Can you work these out from the drawing? Everything is in mm from the part's minimum corner. A direction names the side the tool comes from. Round coordinates to 2 decimals unless told otherwise and drop trailing zeros. Write each loop counter-clockwise with the first axis right and the second up, starting at its lowest first coordinate (ties: lowest second). Pieces come first, ordered by that corner, then holes. Notation, with made-up numbers: (43.25, 80) -> (72.25, 80) arc R17 cw to (72.25, 94) -> close; hole circle Ø9 at (66, 76.25). An arc over 180 degrees is marked (long way). Write item = value, one per line. Start each with the question number.
1) Imagine slicing it at A-A, the plane y = 15. Please give me the cut outline in (x, z).
2) Imagine slicing it at C-C, the plane z = 36.5. Please give me the cut outline in (x, y).
3) If I drill on line 1 (Z direction, x = 5.5, y = 2.25); line 2 (Z direction, x = 10.25, y = 6.5); line 3 (Y direction, x = 16.25, z = 31.5), over which ranges is the centre line in solid material (lowest first)?
4) Imagine slicing it at B-B, the plane x = 15. Please give me the cut outline in (y, z).
5) Imagine slicing it at D-D, the plane x = 7.75. Please give me the cut outline in (y, z), then the cut area to 3 significant figures.
6) For the marked faces 1, 2 and 3, which set-ups out of +Z, -Z, +X, -X, +Y, -Y let a thin tool reach every point of the face, with its end or its side?
7) I'm going to push flat-ended pins straight in: pin 1 (1.2 mm diameter, centred on x = 8, z = 48, fed in from +Y); pin 2 (6 mm diameter, centred on x = 10.5, z = 15.5, fed in from -Y); pin 3 (12 mm diameter, centred on y = 18.5, z = 13.5, fed in from -X). Where does each tip first touch, or does it pass through?
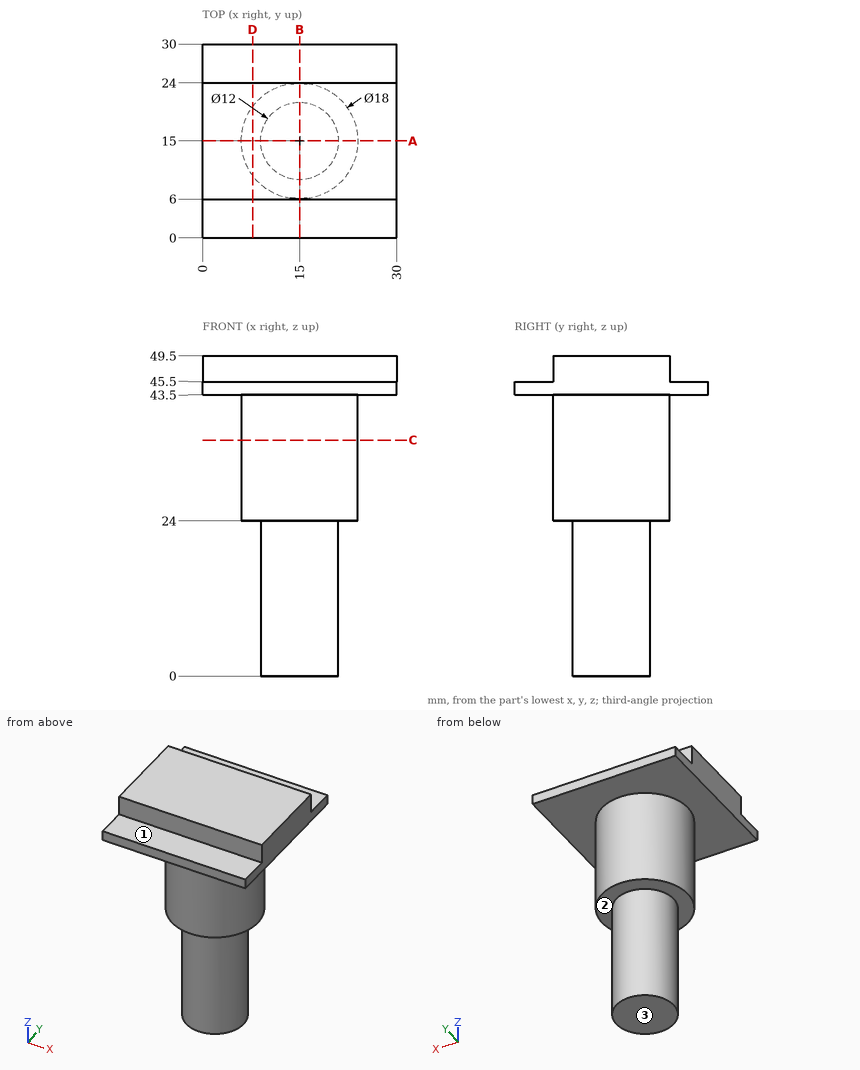
Reported:
q1.outline = (0, 43.5) -> (6, 43.5) -> (6, 24) -> (9, 24) -> (9, 0) -> (21, 0) -> (21, 24) -> (24, 24) -> (24, 43.5) -> (30, 43.5) -> (30, 49.5) -> (0, 49.5) -> close
q2.outline = circle Ø18 at (15, 15)
q3.line_1 = 43.5 to 45.5
q3.line_2 = 43.5 to 49.5
q3.line_3 = 6.09 to 23.91
q4.outline = (0, 43.5) -> (6, 43.5) -> (6, 24) -> (9, 24) -> (9, 0) -> (21, 0) -> (21, 24) -> (24, 24) -> (24, 43.5) -> (30, 43.5) -> (30, 45.5) -> (24, 45.5) -> (24, 49.5) -> (6, 49.5) -> (6, 45.5) -> (0, 45.5) -> close
q5.outline = (0, 43.5) -> (9.67, 43.5) -> (9.67, 24) -> (20.33, 24) -> (20.33, 43.5) -> (30, 43.5) -> (30, 45.5) -> (24, 45.5) -> (24, 49.5) -> (6, 49.5) -> (6, 45.5) -> (0, 45.5) -> close
q5.area = 340 mm²
q6.face_1 = +Z, +X, -X, -Y
q6.face_2 = -Z
q6.face_3 = -Z, +X, -X, +Y, -Y
q7.pin_1 = 24
q7.pin_2 = 9.19
q7.pin_3 = 9
